```python
from build123d import *

# Parameters (mm, degrees)
F0_R     = 1.5
F1_DEPTH = 6


with BuildPart() as f1:
    # F0 (on Front) → F1 (new body, symmetric)
    with BuildSketch(Plane.XZ):
        with BuildLine():
            ThreePointArc((-98.8636363636, 208.62745079), (-438.2123939781, 94.2657898945), (-286.1842105263, -229.961908203))
            ThreePointArc((-286.1842105263, -229.961908203), (0, -271.7872906904), (286.1842105263, -229.961908203))
            ThreePointArc((286.1842105263, -229.961908203), (438.2123939781, 94.2657898945), (98.8636363636, 208.62745079))
            ThreePointArc((98.8636363636, 208.62745079), (0, 182.4836597817), (-98.8636363636, 208.62745079))
        make_face()
        with Locations((-313.5, -49)):
            Circle(F0_R, mode=Mode.SUBTRACT)
        with Locations((94.5, -84)):
            Circle(F0_R, mode=Mode.SUBTRACT)
        with Locations((189.5, -84)):
            Circle(F0_R, mode=Mode.SUBTRACT)
        with Locations((-313.5, 46)):
            Circle(F0_R, mode=Mode.SUBTRACT)
        with Locations((-313.5, 78)):
            Circle(F0_R, mode=Mode.SUBTRACT)
        with Locations((-217.5, 0)):
            Circle(F0_R, mode=Mode.SUBTRACT)
        with Locations((-62, 78)):
            Circle(F0_R, mode=Mode.SUBTRACT)
        with Locations((217.5, 0)):
            Circle(F0_R, mode=Mode.SUBTRACT)
        with Locations((189.5, 78)):
            Circle(F0_R, mode=Mode.SUBTRACT)
    extrude(amount=F1_DEPTH, both=True)


solid = f1.part
```
Part model, mm, in its own coordinate system. Give positions to 0.01 mm unless a question says otherwise; leave off trailing zeros. Write each loop counter-clockwise with the first axis right and the second up, starting at its lowest first coordinate (ties: lowest second). Pieces come first, ordered by that corner, then holes. Notation, with made-up numbers: M 45.5,-8 L 104.5,-8 A17 ccw 104.5,12 Z; hole C 21.5,7 d6. An arc over 180 degrees is marked long. Use CSV: the item, a comma, the result in double quotes.
Item 1: Pin check, flat tips, straight feed: P1, Ø2.5, axis at x = -313.5, z = 78, coming from the -Y side; P2, Ø6, axis at x = 190.5, y = -1.5, coming from the +Z side; P3, Ø3, axis at y = -2, z = -104, coming from the -X side; P4, Ø6, axis at x = 129.5, y = 1.5, coming from the +Z side. Stop position of each tip, or through.
Taken from the geometry:
P1,"passes through"
P2,"stops at z = 238.8"
P3,"stops at x = -434.51"
P4,"stops at z = 224.44"
Item 2: Slice it at A-A on y = -3.5. State how many separate pieces and enclosed holes the cut face has, plus the area to 3 significant figures.
Taken from the geometry:
separate pieces,"1"
enclosed holes,"9"
area,"388,000 mm²"
Item 3: Slice it at C-C on z = 94.5. Write the cut outline in (x, y).
Taken from the geometry:
outline,"M -438.11,-6 L 438.11,-6 L 438.11,6 L -438.11,6 Z"
Item 4: Slice it at B-B on x = -130. Write the cut outline in (y, z).
Taken from the geometry:
outline,"M -6,-263.3 L 6,-263.3 L 6,223.48 L -6,223.48 Z"
Item 5: Drill centre lines: probe 1 along X at (y, z) = (3, -84); probe 2 along X at (y, z) = (-0.75, 78); probe 3 along Z at (x, y) = (94.5, 0.5). Where is each one in solid material? Low to high.
Taken from the geometry:
probe 1,"x = -442.32 to 93, 96 to 188, 191 to 442.32"
probe 2,"x = -444.47 to -315, -312 to -63.5, -60.5 to 188, 191 to 444.47"
probe 3,"z = -267.31 to -85.5, -82.5 to 206.22"
